The model under review builds one solid part; all positions refer to its coordinate system, in mm. Face numbers are marked on the shaded views. A direction names the side the tool comes from. Round coordinates to 2 decimals unless told otherwise and drop trailing zeros. Order: outer loops, then holes, each group sorted by start corner. A loop starts at its lowest first (then second) coordinate and runs counter-clockwise, first axis right, second up. Notation, with made-up numbers: M -9,-0.5 L 47,-0.5 A17 ccw 47,18.5 Z; hole C 59.25,18.25 d1. An arc over 180 degrees is marked long. Answer as a JSON object with one key per item and string values. Group by question number.
1. Add section D-D on y = 6.25. State the section outline as (x, z) points.
2. Add section B-B on z = -5. State the section outline as (x, y) points, and give its area (3 significant figures).
3. Clearance check with flat-ended pins moving along their axes: P1, Ø1, axis at y = 2.5, z = -5, coming from the +X side; P2, Ø1, axis at x = 24, z = -4.5, coming from the +Y side; P3, Ø3, axis at y = 5.5, z = -8, coming from the -X side; P4, Ø4.5, axis at x = 10, z = -5, coming from the -Y side. State where each tip first meets the part, or that it passes through.
4. Add section C-C on x = 29. State the section outline as (y, z) points, and give its area (3 significant figures).
5. Machinability: for the marked faces 1, 2, 3 and 4, which of the approach directions +Z, -Z, +X, -X, +Y, -Y give a long, thin tool a straight path to every point of the face, cutting with its end or side? Answer none if there is none.
6. To check wall thickness, follow probe 1 along X at (y, z) = (4.25, -1); probe 2 along X at (y, z) = (-0.2, -5); probe 3 along Y at (x, z) = (31.5, -0.5). State the ranges of each line that lie inside material, in increasing order. Write a range as [from, to].
7. Add section A-A on x = 10. State the section outline as (y, z) points, and give its area (3 significant figures).
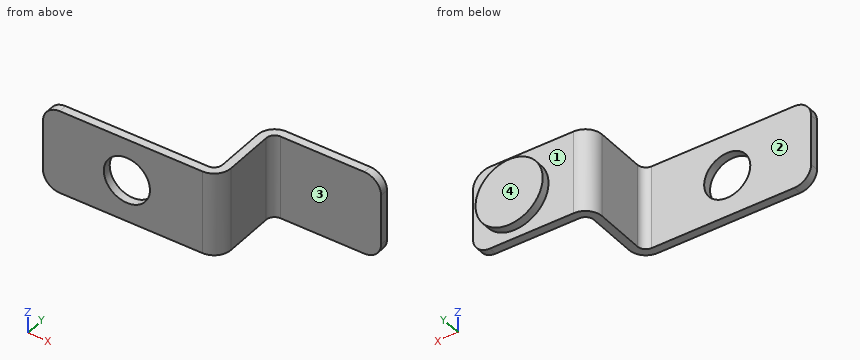
```python
from build123d import *
from build123d.topology import SkipClean

# Parameters (mm, degrees)
SKETCH1_R           = 2.75
BASE_FLANGE1_DEPTH  = 1
JOG1_START          = -10
JOG1_DEPTH          = 10
JOG1_START_2        = -8
JOG1_2_DEPTH        = 6
JOG1_START_3        = 7
JOG1_3_DEPTH        = 1.974011807
JOG1_4_OUTLINE_W    = 1
JOG1_4_OUTLINE_H    = 2
JOG1_4_DEPTH        = 7.152182036
JOG1_START_4        = 8
JOG1_5_DEPTH        = 1
JOG1_6_DEPTH        = 10
JOG1_7_DEPTH        = 10
SKETCH12_R          = 4
BOSS_EXTRUDE1_DEPTH = 1


with BuildPart() as part:
    # Base-Flange1: sheet metal written as solids
    # Sketch1 → Base-Flange1 (new body)
    with BuildSketch(Plane(origin=(0, 0, 0), x_dir=(1, 0, 0), z_dir=(0, 1, 0))):
        with BuildLine():
            Line((0, 2), (0, 8))
            ThreePointArc((0, 8), (0.585786438, 9.414213562), (2, 10))
            Line((2, 10), (32, 10))
            ThreePointArc((32, 10), (33.414213562, 9.414213562), (34, 8))
            Line((34, 8), (34, 2))
            ThreePointArc((34, 2), (33.414213562, 0.585786438), (32, 0))
            Line((32, 0), (2, 0))
            ThreePointArc((2, 0), (0.585786438, 0.585786438), (0, 2))
        make_face()
        with Locations(Location((10, 5, 0), (0, 0, 270))):
            Circle(SKETCH1_R, mode=Mode.SUBTRACT)
    extrude(amount=-BASE_FLANGE1_DEPTH)

    # Jog1: read off the stored shape, not the designer's step
    # Jog1 outline → Jog1 (cut)
    with BuildSketch(Plane.XY.offset(JOG1_START)):
        with BuildLine():
            Line((34, 0), (20.732050807, 0))
            ThreePointArc((20.732050807, 0), (20, -0.732050807), (19, -1))
            Line((19, -1), (34, -1))
            Line((34, -1), (34, 0))
        make_face()
    extrude(amount=JOG1_DEPTH, mode=Mode.SUBTRACT)

    # Jog1 2 outline → Jog1 2 (add)
    with BuildSketch(Plane.XY.offset(JOG1_START_2)):
        with BuildLine():
            Line((21, 1), (21, 7))
            ThreePointArc((21, 7), (21.292893219, 7.707106781), (22, 8))
            Line((22, 8), (34, 8))
            Line((34, 8), (34, 9))
            Line((34, 9), (22, 9))
            ThreePointArc((22, 9), (20.585786438, 8.414213562), (20, 7))
            Line((20, 7), (20, 1))
            ThreePointArc((20, 1), (19.707106781, 0.292893219), (19, 0))
            Line((19, 0), (20.732050807, 0))
            ThreePointArc((20.732050807, 0), (20.931851652, 0.48236191), (21, 1))
        make_face()
    extrude(amount=JOG1_2_DEPTH)

    # Jog1 3 outline → Jog1 3 (add)
    with BuildSketch(Plane(origin=(0, 0, 0), x_dir=(1, 0, 0), z_dir=(0, 1, 0)).offset(JOG1_START_3)):
        with BuildLine():
            Line((20, 10), (20, 8))
            Line((20, 8), (34, 8))
            ThreePointArc((34, 8), (33.414213562, 9.414213562), (32, 10))
            Line((32, 10), (20, 10))
        make_face()
        with BuildLine():
            Line((34, 2), (20, 2))
            Line((20, 2), (20, 0))
            Line((20, 0), (32, 0))
            ThreePointArc((32, 0), (33.414213562, 0.585786438), (34, 2))
        make_face()
    extrude(amount=JOG1_3_DEPTH)

    # Jog1 4 outline → Jog1 4 (add)
    with BuildSketch(Plane(origin=(0, 0, 0), x_dir=(1, 0, 0), z_dir=(0, 1, 0))):
        with Locations((20.5, 9)):
            Rectangle(JOG1_4_OUTLINE_W, JOG1_4_OUTLINE_H)
        with Locations((20.5, 1)):
            Rectangle(JOG1_4_OUTLINE_W, JOG1_4_OUTLINE_H)
    extrude(amount=JOG1_4_DEPTH)

    # Jog1 5 outline → Jog1 5 (add)
    with BuildSketch(Plane(origin=(0, 0, 0), x_dir=(1, 0, 0), z_dir=(0, 1, 0)).offset(JOG1_START_4)):
        with BuildLine():
            Line((32, 10), (21, 10))
            Line((21, 10), (21, 8))
            Line((21, 8), (34, 8))
            ThreePointArc((34, 8), (33.414213562, 9.414213562), (32, 10))
        make_face()
        with BuildLine():
            Line((34, 2), (21, 2))
            Line((21, 2), (21, 0))
            Line((21, 0), (32, 0))
            ThreePointArc((32, 0), (33.414213562, 0.585786438), (34, 2))
        make_face()
    extrude(amount=JOG1_5_DEPTH)

    # Jog1 6 outline → Jog1 6 (cut)
    with SkipClean():  # the faces are left unmerged after this step: merging them gives an invalid solid
        with BuildSketch(Plane.XY.offset(JOG1_START)):
            with BuildLine():
                Line((21, 7), (21, 1))
                ThreePointArc((21, 1), (20.732050807, -1e-09), (19.999999998, -0.732050808))
                Line((19.999999998, -0.732050808), (19.999999995, -1))
                Line((19.999999995, -1), (35, -1))
                Line((35, -1), (35, 8))
                Line((35, 8), (22, 8))
                ThreePointArc((22, 8), (21.292893219, 7.707106781), (21, 7))
            make_face()
            with BuildLine():
                Line((21, 9), (21, 8.974011807))
                Line((21, 8.974011807), (20, 8.974011807))
                Line((20, 8.974011807), (20, 7))
                ThreePointArc((20, 7), (20.585786438, 8.414213562), (22, 9))
                Line((22, 9), (35, 9.000000008))
                Line((35, 9.000000008), (35, 10))
                Line((35, 10), (21.000000006, 10))
                Line((21.000000006, 10), (21, 9))
            make_face()
        extrude(amount=JOG1_6_DEPTH, mode=Mode.SUBTRACT)
    add(part.part.scale(1), mode=Mode.REPLACE)  # the faces are merged on a copy

    # Jog1 7 outline → Jog1 7 (add)
    with BuildSketch(Plane.XY.offset(JOG1_START)):
        with BuildLine():
            ThreePointArc((19, -1), (19.517638089, -0.931851653), (19.999999998, -0.732050808))
            Line((19.999999998, -0.732050808), (19.999999996, 0))
            Line((19.999999996, 0), (20, 1))
            ThreePointArc((20, 1), (19.707106781, 0.292893219), (19, 0))
            Line((19, 0), (18, -1e-09))
            Line((18, -1e-09), (18, -1))
            Line((18, -1), (19, -1))
        make_face()
    extrude(amount=JOG1_7_DEPTH)

    # Sketch12 → Boss-Extrude1 (add)
    with BuildSketch(Plane(origin=(0, 9, 0), x_dir=(1, 0, 0), z_dir=(0, 1, 0))):
        with Locations(Location((29, 5, 0), (0, 0, 180))):
            Circle(SKETCH12_R)
    extrude(amount=BOSS_EXTRUDE1_DEPTH)


solid = part.part
```
Recorded:
{
 "1": {"outline": "M 20,-10 L 21,-10 L 21,0 L 20,0 Z"},
 "2": {"outline": "M 0,-1 L 7.25,-1 L 7.25,0 L 0,0 Z; M 12.75,-1 L 19,-1 A2 ccw 21,1 L 21,7 A1 cw 22,8 L 34,8 L 34,9 L 33,9 L 33,10 L 25,10 L 25,9 L 22,9 A2 ccw 20,7 L 20,1 A1 cw 19,0 L 12.75,0 Z", "area": "44.2 mm²"},
 "3": {"P1": "stops at x = 21", "P2": "stops at y = 9", "P3": "stops at x = 20", "P4": "passes through"},
 "4": {"outline": "M 8,-10 L 9,-10 L 9,-9 L 10,-9 L 10,-1 L 9,-1 L 9,0 L 8,0 Z", "area": "18.0 mm²"},
 "5": {"face 1": "+Y", "face 2": "+Z, -Z, -X, +Y", "face 3": "+Z, -Z, +X, -Y", "face 4": "+Z, -Z, +X, -X, +Y"},
 "6": {"probe 1": "x = [20, 21]", "probe 2": "x = [0, 7.25], [12.75, 20.6]", "probe 3": "y = [8, 9]"},
 "7": {"outline": "M -1,-10 L 0,-10 L 0,-7.75 L -1,-7.75 Z; M -1,-2.25 L 0,-2.25 L 0,0 L -1,0 Z", "area": "4.50 mm²"}
}
